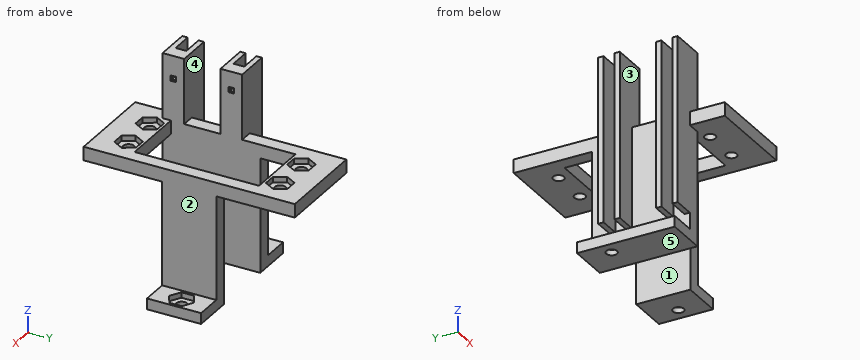
from build123d import *

# Parameters (mm, degrees)
SKETCH1_W                     = 17
SKETCH1_H                     = 39
SKETCH1_R                     = 1
SKETCH1_W_2                   = 12
SKETCH1_H_2                   = 23
SERVOBRACKET_DEPTH            = 2.5
SKETCH1_5_W                   = 2.5
SKETCH1_5_H                   = 10
SUPPORTLEGS_DEPTH             = 21.1
SKETCH2_W                     = 2
SKETCH2_H                     = 10
SUPPORTFOOT_DEPTH             = 5
BASEBOLTHOLE_START            = -3
SKETCH3_R                     = 1
BASEBOLTHOLE_DEPTH            = 25.6
SERVONUTSLOTS_DEPTH           = 1
BASENUTSLOTS_DEPTH            = 1
SKETCH6_W                     = 2.5
SKETCH6_H                     = 4
TUBEHOLDERBASE_DEPTH          = 12
SKETCH7_W                     = 4
SKETCH7_H                     = 1
TUBEHOLDERSTIFFENERRIBS_DEPTH = 30.6
SKETCH8_W                     = 1
SKETCH8_H                     = 1
SKETCH8_W_2                   = 1.5
SKETCH8_H_2                   = 1.5
TUBECLIPENTRANCES_DEPTH       = 2
SKETCH8_3_W                   = 1
SKETCH8_3_H                   = 1
CABLEEXITS_DEPTH              = 2.5
SKETCH9_W                     = 1.5
SKETCH9_H                     = 1.5
TUBECLIPLOCKSLOT_DEPTH        = 0.6
SKETCH10_W                    = 1.5
SKETCH10_H                    = 1.5
TUBECLIPLOCKSLOT2_DEPTH       = 0.6
SUPPORTLEGEXTENSION_DEPTH     = 8.05
SKETCH8_4_W                   = 0.2
SKETCH8_4_H                   = 1.5
TUBECLIPLOCKCLEARANCE_DEPTH   = 0.5


with BuildPart() as part:
    # Sketch1 → ServoBracket (new body)
    with BuildSketch(Plane.XY):
        with Locations((0, 19.5)):
            Rectangle(SKETCH1_W, SKETCH1_H)
        with Locations((-3.5, 33.5)):
            Circle(SKETCH1_R, mode=Mode.SUBTRACT)
        with Locations((-3.5, 5.5)):
            Circle(SKETCH1_R, mode=Mode.SUBTRACT)
        with Locations((3.5, 5.5)):
            Circle(SKETCH1_R, mode=Mode.SUBTRACT)
        with Locations((3.5, 33.5)):
            Circle(SKETCH1_R, mode=Mode.SUBTRACT)
        with Locations((0, 19.5)):
            Rectangle(SKETCH1_W_2, SKETCH1_H_2, mode=Mode.SUBTRACT)
    extrude(amount=SERVOBRACKET_DEPTH)

    # Sketch1<5> → SupportLegs (add)
    with BuildSketch(Plane.XY):
        with Locations((-7.25, 19.5)):
            Rectangle(SKETCH1_5_W, SKETCH1_5_H)
        with Locations((7.25, 19.5)):
            Rectangle(SKETCH1_5_W, SKETCH1_5_H)
    extrude(amount=-SUPPORTLEGS_DEPTH)

    # Sketch2 → SupportFoot (add)
    with BuildSketch(Plane.ZY.offset(8.5)):
        with Locations((-20.1, 19.5)):
            Rectangle(SKETCH2_W, SKETCH2_H)
    supportfoot = extrude(amount=SUPPORTFOOT_DEPTH)

    # Sketch3 → BaseBoltHole (cut)
    with BuildSketch(Plane.XY.offset(-19.1).offset(BASEBOLTHOLE_START)):
        with Locations((-11, 19.5)):
            Circle(SKETCH3_R)
    basebolthole = extrude(amount=BASEBOLTHOLE_DEPTH, mode=Mode.SUBTRACT)

    # SupportFoot2: SupportFoot, BaseBoltHole across plane
    add(supportfoot.mirror(Plane(origin=(0, 0, 0), x_dir=(0, 0, 1), z_dir=(1, 0, 0))))
    add(basebolthole.mirror(Plane(origin=(0, 0, 0), x_dir=(0, 0, 1), z_dir=(1, 0, 0))), mode=Mode.SUBTRACT)

    # Sketch4 → ServoNutSlots (cut)
    with BuildSketch(Plane.XY.offset(2.5)):
        Polygon((-4.654700538, 7.5), (-2.345299462, 7.5), (-1.190598923, 5.5), (-2.345299462, 3.5), (-4.654700538, 3.5), (-5.809401077, 5.5), align=None)
        Polygon((-1.190598923, 33.5), (-2.345299462, 35.5), (-4.654700538, 35.5), (-5.809401077, 33.5), (-4.654700538, 31.5), (-2.345299462, 31.5), align=None)
        Polygon((2.345299462, 31.5), (1.190598923, 33.5), (2.345299462, 35.5), (4.654700538, 35.5), (5.809401077, 33.5), (4.654700538, 31.5), align=None)
        Polygon((4.654700538, 7.5), (2.345299462, 7.5), (1.190598923, 5.5), (2.345299462, 3.5), (4.654700538, 3.5), (5.809401077, 5.5), align=None)
    extrude(amount=-SERVONUTSLOTS_DEPTH, mode=Mode.SUBTRACT)

    # Sketch5 → BaseNutSlots (cut)
    with BuildSketch(Plane.XY.offset(-19.1)):
        Polygon((-11, 21.809401077), (-13, 20.654700538), (-13, 18.345299462), (-11, 17.190598923), (-9, 18.345299462), (-9, 20.654700538), align=None)
        Polygon((11, 21.809401077), (9, 20.654700538), (9, 18.345299462), (11, 17.190598923), (13, 18.345299462), (13, 20.654700538), align=None)
    extrude(amount=-BASENUTSLOTS_DEPTH, mode=Mode.SUBTRACT)

    # Sketch6 → TubeHolderBase (add)
    with BuildSketch(Plane.XY.offset(2.5)):
        with Locations((-7.25, 19.15)):
            Rectangle(SKETCH6_W, SKETCH6_H)
    tubeholderbase = extrude(amount=TUBEHOLDERBASE_DEPTH)

    # Sketch7 → TubeHolderStiffenerRibs (add)
    with BuildSketch(Plane.XY.offset(14.5)):
        with Locations((-10.5, 20.65)):
            Rectangle(SKETCH7_W, SKETCH7_H)
        with Locations((-10.5, 17.65)):
            Rectangle(SKETCH7_W, SKETCH7_H)
    tubeholderstiffenerribs = extrude(amount=-TUBEHOLDERSTIFFENERRIBS_DEPTH)

    # TubeHolder2: TubeHolderBase, TubeHolderStiffenerRibs across plane
    add(tubeholderbase.mirror(Plane.ZX.offset(13.8)))
    add(tubeholderstiffenerribs.mirror(Plane.ZX.offset(13.8)))

    # Sketch8 → TubeClipEntrances (cut)
    with BuildSketch(Plane.ZY.offset(8.5)):
        with Locations((11.1, 19.15)):
            Rectangle(SKETCH8_W, SKETCH8_H)
        with Locations((11.1, 19.15)):
            Rectangle(SKETCH8_W_2, SKETCH8_H_2)
        with Locations((11.1, 19.15)):
            Rectangle(SKETCH8_W, SKETCH8_H, mode=Mode.SUBTRACT)
        with Locations((10.3, 8.45)):
            Rectangle(SKETCH8_W, SKETCH8_H)
        with Locations((10.3, 8.45)):
            Rectangle(SKETCH8_W_2, SKETCH8_H_2)
        with Locations((10.3, 8.45)):
            Rectangle(SKETCH8_W, SKETCH8_H, mode=Mode.SUBTRACT)
    extrude(amount=-TUBECLIPENTRANCES_DEPTH, mode=Mode.SUBTRACT)

    # Sketch8<3> → CableExits (cut)
    with BuildSketch(Plane.ZY.offset(8.5)):
        with Locations((11.1, 19.15)):
            Rectangle(SKETCH8_3_W, SKETCH8_3_H)
        with Locations((10.3, 8.45)):
            Rectangle(SKETCH8_3_W, SKETCH8_3_H)
    extrude(amount=-CABLEEXITS_DEPTH, mode=Mode.SUBTRACT)

    # Sketch9 → TubeClipLockSlot (cut)
    with BuildSketch(Plane(origin=(0, 0, 11.85), x_dir=(-1, 0, 0), z_dir=(0, 0, -1))):
        with Locations((7.25, 19.15)):
            Rectangle(SKETCH9_W, SKETCH9_H)
    extrude(amount=-TUBECLIPLOCKSLOT_DEPTH, mode=Mode.SUBTRACT)

    # Sketch10 → TubeClipLockSlot2 (cut)
    with BuildSketch(Plane(origin=(0, 0, 11.05), x_dir=(-1, 0, 0), z_dir=(0, 0, -1))):
        with Locations((7.25, 8.45)):
            Rectangle(SKETCH10_W, SKETCH10_H)
    extrude(amount=-TUBECLIPLOCKSLOT2_DEPTH, mode=Mode.SUBTRACT)

    # Sketch11 → SupportLegExtension (add)
    with BuildSketch(Plane.XZ.offset(-14.5)):
        Polygon((-6, 0), (-8.5, 0), (-8.5, -19.1), (-13.5, -19.1), (-13.5, -21.1), (-6, -21.1), align=None)
    extrude(amount=SUPPORTLEGEXTENSION_DEPTH)

    # Sketch8<4> → TubeClipLockClearance (cut)
    with BuildSketch(Plane.ZY.offset(8.5)):
        with Locations((11.15, 8.45)):
            Rectangle(SKETCH8_4_W, SKETCH8_4_H)
        with Locations((11.95, 19.15)):
            Rectangle(SKETCH8_4_W, SKETCH8_4_H)
    extrude(amount=-TUBECLIPLOCKCLEARANCE_DEPTH, mode=Mode.SUBTRACT)


solid = part.part
Design review of the part built by this model. Coordinates are the model's own, in mm. Face numbers are marked on the shaded views. A direction names the side the tool comes from. Give positions to 0.01 mm unless a question says otherwise; leave off trailing zeros. Loops run counter-clockwise (first coordinate to the right, second up) from the corner with the lowest first, then second, coordinate; pieces in that order, holes last. Notation, with made-up numbers: (73, 47.5) - (95, 47.5) arc R18 cw to (95, 70.5) - close; hole circle Ø2 at (43, 38). An arc over 180 degrees is marked (long way). Use CSV: the item, a comma, the result in double quotes. Start each with the question number.
1. Draft analysis for pull direction Y (two halves, no side actions). For the marked faces 4 and 5, state which applies: released by +Y, released by -Y, zero draft, split by the parting line, or undercut.
2. Add section A-A (y = 15.5). State the section outline as (x, z) points, plus the area to 3 significant figures.
3. Insertion check: P1, Ø1.5, axis at x = -8.5, y = 22, coming from the +Z side; P2, Ø0.5, axis at y = 10, z = -2.5, coming from the -X side; P3, Ø1, axis at x = -7.5, z = 11, coming from the -Y side; P4, Ø1.5, axis at x = -3.5, z = 8, coming from the -Y side. Each pin has a flat end and moves straight along its axis. Give the tip position at first contact, or say it passes through.
4. Add section B-B (z = -17.5). State the section outline as (x, y) points.
5. Add section D-D (x = -3.5). State the section outline as (y, z) points.
6. Add section C-C (x = 0). State the section outline as (y, z) points.
7. Machinability: for the marked faces 1, 2 and 3, which of the approach directions +Z, -Z, +X, -X, +Y, -Y give a long, thin tool a straight path to every point of the face, cutting with its end or side? Answer none if there is none.
8. Wall thickness on L1, parallel to Y at x = -3.5, z = 0.8; L2, parallel to X at y = 33.5, z = 1.15; L3, parallel to Y at x = 2.25, z = 2: over which ranges is each line inside the solid? List them lowest first.
Results found:
1,face 4,"undercut"
1,face 5,"zero draft"
2,outline,"(-13.5, -21.1) - (-6, -21.1) - (-6, 2.5) - (-8.5, 2.5) - (-8.5, -19.1) - (-13.5, -19.1) - close; (6, -21.1) - (13.5, -21.1) - (13.5, -19.1) - (8.5, -19.1) - (8.5, 2.5) - (6, 2.5) - close"
2,area,"138 mm²"
3,P1,"stops at z = 2.5"
3,P2,"stops at x = -12.5"
3,P3,"stops at y = 6.45"
3,P4,"passes through"
4,outline,"(-8.5, 6.45) - (-6, 6.45) - (-6, 24.5) - (-8.5, 24.5) - close; (6, 14.5) - (8.5, 14.5) - (8.5, 24.5) - (6, 24.5) - close"
5,outline,"(0, 0) - (4.5, 0) - (4.5, 1.5) - (3.5, 1.5) - (3.5, 2.5) - (0, 2.5) - close; (6.5, 0) - (8, 0) - (8, 2.5) - (7.5, 2.5) - (7.5, 1.5) - (6.5, 1.5) - close; (31, 0) - (32.5, 0) - (32.5, 1.5) - (31.5, 1.5) - (31.5, 2.5) - (31, 2.5) - close; (34.5, 0) - (39, 0) - (39, 2.5) - (35.5, 2.5) - (35.5, 1.5) - (34.5, 1.5) - close"
6,outline,"(0, 0) - (8, 0) - (8, 2.5) - (0, 2.5) - close; (31, 0) - (39, 0) - (39, 2.5) - (31, 2.5) - close"
7,face 1,"+Z, -Z"
7,face 2,"+Z, +X, +Y, -Y"
7,face 3,"+Z, -X"
8,L1,"y = 0 to 4.5, 6.5 to 8, 31 to 32.5, 34.5 to 39"
8,L2,"x = -8.5 to -4.5, -2.5 to 2.5, 4.5 to 8.5"
8,L3,"y = 0 to 3.67, 7.33 to 8, 31 to 31.67, 35.33 to 39"
